Geometry check sheet. Reference: the model listing, model coordinates, mm. Coordinates: 2 decimals unless noted, no trailing zeros. Loops run counter-clockwise (first coordinate to the right, second up) from the corner with the lowest first, then second, coordinate; pieces in that order, holes last.
Autodesk Fusion 360 part; units mm, degrees
sketch "Sketch1" plane through (0, 0, 0) normal (0, 1, 0) x (1, 0, 0)
  circle A0 centre (0, 0) radius 14 construction
  line L0 (0, 0) -> (0, 52) construction
  circle A1 centre (0, 0) radius 58 construction
  line L1 (0, 0) -> (-58, 0) construction
  line L2 (-61.5, 0) -> (-54.5, 0) construction
  line L3 (-52.0547, 32.75) -> (-43.5625, 32.75) construction
  line L4 (-54.7818, 27.95) -> (-46.7873, 27.95) construction
  line L5 (-59.0893, -17.05) -> (-51.7643, -17.05) construction
  circle A2 centre (-57.1227, -10.05) radius 1.5
  circle A3 centre (-54.0842, 20.95) radius 1.5
  arc A4 (-50.8205, 19.6858) -> (-57.3479, 22.2142) centre (-54.0842, 20.95) ccw
  arc A5 (-57.3479, 22.2142) -> (-55.2493, 17.6496) centre (-54.0842, 20.95) ccw construction
  arc A6 (-55.2493, 17.6496) -> (-50.8205, 19.6858) centre (-54.0842, 20.95) ccw construction
  arc A7 (-60.5697, -10.6565) -> (-53.6756, -9.4435) centre (-57.1227, -10.05) ccw
  arc A8 (-57.6248, -6.5862) -> (-60.5697, -10.6565) centre (-57.1227, -10.05) ccw construction
  arc A9 (-53.6756, -9.4435) -> (-57.6248, -6.5862) centre (-57.1227, -10.05) ccw construction
  arc A10 (-60.5697, -10.6565) -> (-59.0893, -17.05) centre (0, 0) ccw construction
  arc A11 (-53.6756, -9.4435) -> (-51.7643, -17.05) centre (0, 0) ccw construction
  arc A12 (-51.7643, -17.05) -> (-46.7873, 27.95) centre (0, 0) ccw construction
  arc A13 (-50.8205, 19.6858) -> (-53.6756, -9.4435) centre (0, 0) ccw
  arc A14 (-46.7873, 27.95) -> (-50.8205, 19.6858) centre (0, 0) ccw construction
  arc A15 (-59.0893, -17.05) -> (-54.7818, 27.95) centre (0, 0) ccw construction
  arc A16 (-57.3479, 22.2142) -> (-60.5697, -10.6565) centre (0, 0) ccw
  arc A17 (-54.7818, 27.95) -> (-57.3479, 22.2142) centre (0, 0) ccw construction
  point P0 (0, 14)
  point P1 (-58, 0)
  point P2 (-54.0842, 20.95)
  point P3 (-57.1227, -10.05)
  dimension "d6" = 28
  dimension "d7" = 38
  dimension "d8" = 116
  dimension "d9" = 7
  dimension "d10" = 19.25
  dimension "d11" = 4.8
  dimension "d12" = 7
  dimension "d13" = 45
  dimension "d14" = 7
  dimension "d15" = 3
  dimension "d16" = 3
extrude "Extrude1" add sketch "Sketch1" along normal blind 4.8
(1) Sectioned sample at B-B on x = -55. Record the cut outline in (y, z).
Findings:
outline: (0, -24.33) - (4.8, -24.33) - (4.8, -22.14) - (0, -22.14) - close; (0, -19.76) - (4.8, -19.76) - (4.8, 12.83) - (0, 12.83) - close
(2) Gauge pin test, flat ends, axial feed: pin 1 Ø1 at (x, y) = (-52.5, 3.5) entering from -Z; pin 2 Ø2 at (y, z) = (3, -17) entering from +X. Record the tip position at first contact, or that the pin passes through.
Findings:
pin 1: stops at z = -24.28
pin 2: stops at x = -51.44
(3) Sectioned sample at A-A on z = 10.05. Record the cut outline in (x, y).
Findings:
outline: (-60.67, 0) - (-58.62, 0) - (-58.62, 4.8) - (-60.67, 4.8) - close; (-55.62, 0) - (-53.62, 0) - (-53.62, 4.8) - (-55.62, 4.8) - close
(4) Sectioned sample at C-C on y = 1.8. Record the cut outline in (x, z).
Findings:
outline: (-60.57, 10.66) arc R61.5 ccw to (-57.35, -22.21) arc R3.5 ccw to (-50.82, -19.69) arc R54.5 cw to (-53.68, 9.44) arc R3.5 ccw to start; hole circle Ø3 at (-57.12, 10.05); hole circle Ø3 at (-54.08, -20.95)
(5) Sectioned sample at D-D on x = -52. Record the cut outline in (y, z), and give its area (3 significant figures).
Findings:
outline: (0, -23.76) - (4.8, -23.76) - (4.8, -16.32) - (0, -16.32) - close
area: 35.7 mm2
(6) Draft check along Z on faces 1 (the flat face through (-57, 4.8, -6)), 2 (the cylindrical face through (-61.23, 2.37, -5.77)), 3 (the cylindrical face through (-54.26, 2.37, -5.11)). Enter one of: +Z half, -Z half, draft (parallel to the pull), parting line (faces both ways), or undercut.
Findings:
face 1: draft
face 2: parting line
face 3: undercut
(7) Scan lines: L1, parallel to Z at x = -56.25, y = 3.6; L2, parallel to X at y = 3.55, z = -20.95; L3, parallel to X at y = 3.6, z = 10.05. Record each from-to range of solid material in increasing order.
Findings:
L1: z = -23.7 to 8.83, 11.27 to 13.44
L2: x = -57.82 to -55.58, -52.58 to -50.58
L3: x = -60.67 to -58.62, -55.62 to -53.62
